Autodesk Inventor part; units mm, degrees
ref_plane "YZ Plane" through (0, 0, 0) normal (1, 0, 0) x (0, 1, 0)
ref_plane "XZ Plane" through (0, 0, 0) normal (0, 1, 0) x (-1, 0, 0)
ref_plane "XY Plane" through (0, 0, 0) normal (0, 0, 1) x (1, 0, 0)
sketch "Sketch1" plane through (0, 0, 0) normal (0, 0, 1) x (1, 0, 0)
  line L0 (0, 0) -> (11, 0)
  line L1 (11, 0) -> (11, 2.1)
  line L2 (11, 2.1) -> (0, 2.1)
  line L3 (0, 2.1) -> (0, 0)
  line L4 (0, 0) -> (5, 0)
  line L5 (5, 0) -> (5, 12.1)
  line L6 (5, 12.1) -> (0, 12.1)
  line L7 (0, 12.1) -> (0, 0)
  line L8 (0, 12.1) -> (2, 12.1)
  line L9 (2, 12.1) -> (2, 0)
  line L10 (2, 0) -> (0, 0)
  line L11 (0, 0) -> (0, 12.1)
  point P0 (2, 0)
  point P1 (5, 2.1)
  dimension "d0" = 11
  dimension "d1" = 2.1
  dimension "d2" = 5
  dimension "d3" = 12.1
  dimension "d4" = 2
revolve "Revolution1" add sketch "Sketch1" angle 360 about axis through (0, 12.1, 0) along (0, -1, 0) contours L9 L2 L5 L0 | L5 L2 L1 L0 | L9 L6 L5 L2
sketch "Sketch2" plane through (0, 0, 0) normal (0, -1, 0) x (1, 0, 0)
  circle A0 centre (0, 0) radius 8 construction
  line L0 (0, 0) -> (8, 0) construction
  circle A1 centre (8, 0) radius 1.5
  circle A2 centre (0, 8) radius 1.5
  circle A3 centre (-8, 0) radius 1.5
  circle A4 centre (0, -8) radius 1.5
  dimension "d6" = 16
  dimension "d7" = 3
  dimension "d10" = 360
extrude "Extrusion1" cut sketch "Sketch2" against normal through all
sketch "Sketch3" plane through (0, 0, 0) normal (1, 0, 0) x (0, 1, 0)
  line L0 (12.1, 5) -> (12.1, -5)
  line L1 (12.1, 0) -> (0, 0) construction
  circle A0 centre (9.1, 0) radius 1.25
  dimension "d14" = 2.5
  dimension "d15" = 3
extrude "Extrusion2" cut sketch "Sketch3" along normal through all both and the other way through all
chamfer "Chamfer1" distance 0.5 angle 45 2 edges at (-5, 12.1, 0) (-2, 12.1, 0)
chamfer "Chamfer2" distance 0.25 angle 45 5 edges at (-11, 0, 0) (-11, 2.1, 0) (4.8412, 9.0999, -1.25) (4.8412, 9.1, 1.25) (-5, 7.85, -0.0003)
properties part number "Hubs - 4mm" material "Stainless Steel"
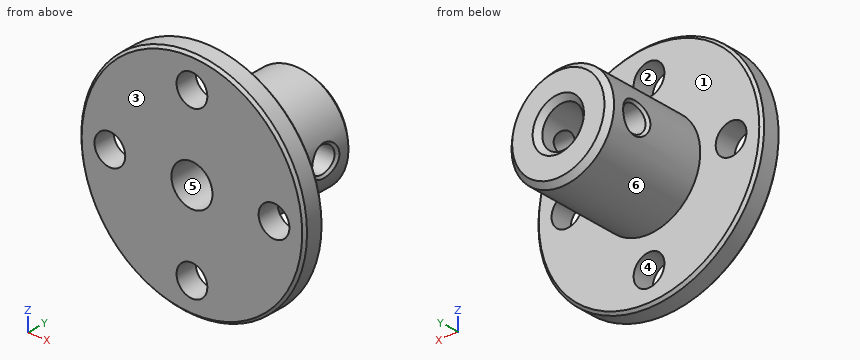
Model file for the job. Use its own axes, mm. Face numbers are marked on the shaded views. A direction names the side the tool comes from. Round coordinates to 2 decimals unless told otherwise and drop trailing zeros. Loops run counter-clockwise (first coordinate to the right, second up) from the corner with the lowest first, then second, coordinate; pieces in that order, holes last.
1. Mould opens along Z. For the marked faces 3, 4, 5 and 6 say: +Z half, -Z half, draft (parallel to the pull), parting line (faces both ways), or undercut.
Check values:
face 3: draft
face 4: undercut
face 5: undercut
face 6: parting line
2. Band-saw the part on A-A, the plane y = 1.25. List the corners of the cut face in (x, z).
Check values:
outline: circle Ø22 at (0, 0); hole circle Ø3 at (-8, 0); hole circle Ø4 at (0, 0); hole circle Ø3 at (0, -8); hole circle Ø3 at (0, 8); hole circle Ø3 at (8, 0)
3. Wall check: probe 1 along X at (y, z) = (3.5, 0); probe 2 along Y at (x, z) = (2.75, 4.5); probe 3 along Z at (x, y) = (-4.1, 9.1). Give the ranges that are in metal, low to high.
Check values:
probe 1: x = -5 to -2, 2 to 5
probe 2: y = 0 to 2.1
probe 3: z = -2.86 to -1.25, 1.25 to 2.86
4. Band-saw the part on C-C, the plane y = 3. List the corners of the cut face in (x, z), and give its area (3 significant figures).
Check values:
outline: circle Ø10 at (0, 0); hole circle Ø4 at (0, 0)
area: 66.0 mm2
5. Band-saw the part on B-B, the plane x = 0. List the corners of the cut face in (y, z), and give its area (3 significant figures).
Check values:
outline: (0, -10.75) - (0.25, -11) - (1.85, -11) - (2.1, -10.75) - (2.1, -9.5) - (0, -9.5) - close; (0, -6.5) - (2.1, -6.5) - (2.1, -5) - (11.6, -5) - (12.1, -4.5) - (12.1, -2.5) - (11.6, -2) - (0, -2) - close; (0, 2) - (11.6, 2) - (12.1, 2.5) - (12.1, 4.5) - (11.6, 5) - (2.1, 5) - (2.1, 6.5) - (0, 6.5) - close; (0, 9.5) - (2.1, 9.5) - (2.1, 10.75) - (1.85, 11) - (0.25, 11) - (0, 10.75) - close
area: 84.6 mm2
6. Drop flat-ended pins along their axis: P1, Ø3.5, axis at x = -8, z = 0, coming from the +Y side; P2, Ø2, axis at y = 7, z = 2, coming from the -X side; P3, Ø1, axis at y = 5.5, z = 2, coming from the -X side. Give the stop position or say it passes through.
Check values:
P1: stops at y = 2.1
P2: stops at x = -4.9
P3: stops at x = -4.77
7. Tool access for the marked faces 1 and 2: list every direction of +Z, -Z, +X, -X, +Y, -Y with a clear straight run to the whole face (end or side of a thin tool).
Check values:
face 1: +Y
face 2: +Y, -Y
